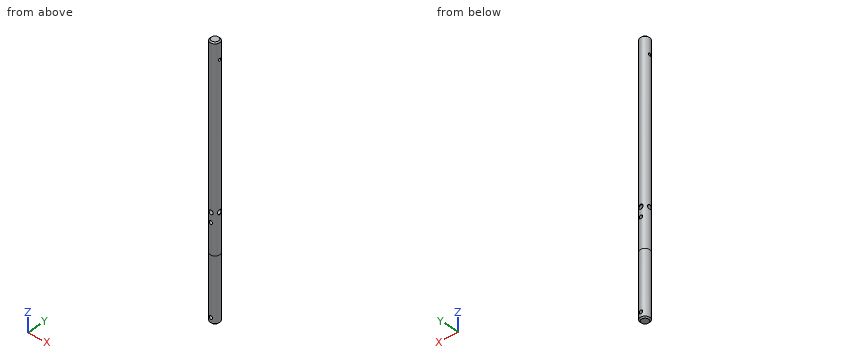
from build123d import *

# Parameters (mm, degrees)
SKETCH1_W                                 = 3.175
SKETCH1_H                                 = 133.223
F_2_56_TAPPED_HOLE1_D                     = 1.778
SKETCH4_R                                 = 3.175
BOSS_EXTRUDE1_DEPTH                       = 43.053
CHAMFER1_SIZE                             = 0.762
F_4_40_TAPPED_HOLE2_D                     = 2.2606
F_7_64_0_10938_DIAMETER_HOLE2_D           = 2.778252
F_7_64_0_10938_DIAMETER_HOLE2_CSINK_D     = 3.175
F_7_64_0_10938_DIAMETER_HOLE2_CSINK_ANGLE = 82


with BuildPart() as part:
    # Sketch1 → Revolve1 (revolve)
    with BuildSketch(Plane.XZ):
        with Locations((1.5875, 66.6115)):
            Rectangle(SKETCH1_W, SKETCH1_H)
    revolve(axis=Axis((0, 0, 133.223), (0, 0, -1)))

    # #2-56 Tapped Hole1 (through all)
    with Locations(Plane(origin=(3.175, 0, 0), x_dir=(0, 0, -1), z_dir=(1, 0, 0))):
        with Locations((-121.801801862, 0)):
            Hole(F_2_56_TAPPED_HOLE1_D / 2)

    # Sketch4 → Boss-Extrude1 (add)
    with BuildSketch(Plane(origin=(0, 0, 0), x_dir=(-1, 0, 0), z_dir=(0, 0, -1))):
        Circle(SKETCH4_R)
    extrude(amount=BOSS_EXTRUDE1_DEPTH)

    # Chamfer1
    chamfer1_edges = [part.edges().sort_by_distance(p)[0] for p in [
        (3.175, 0, -43.053),
        (-3.175, 0, 133.223),
    ]]
    chamfer(chamfer1_edges, length=CHAMFER1_SIZE)

    # #4-40 Tapped Hole2 (through all)
    with Locations(Plane(origin=(0, -3.175, 0), x_dir=(-1, 0, 0), z_dir=(0, -1, 0))):
        with Locations((0, -20.32), (0, 39.0271)):
            Hole(F_4_40_TAPPED_HOLE2_D / 2)

    # Sketch10 → 7/64 (0.10938) Diameter Hole1 (revolve, cut)
    with BuildSketch(Plane(origin=(0, -3.175, 26.67), x_dir=(0, 0, -1), z_dir=(1, 0, 0))):
        Polygon((0, 0), (0, 6.35), (1.5875, 6.35), (1.389126, 6.121796818), (1.389126, 0), align=None)
    revolve(axis=Axis((0, -9.525, 26.67), (0, 1, 0)), mode=Mode.SUBTRACT)

    # 7/64 (0.10938) Diameter Hole2 (through all)
    with Locations(Plane(origin=(3.175, 0, 0), x_dir=(0, 0, -1), z_dir=(1, 0, 0))):
        with Locations((-26.67, 0)):
            CounterSinkHole(F_7_64_0_10938_DIAMETER_HOLE2_D / 2, F_7_64_0_10938_DIAMETER_HOLE2_CSINK_D / 2, counter_sink_angle=F_7_64_0_10938_DIAMETER_HOLE2_CSINK_ANGLE)


solid = part.part
Could you check a few things on this model? Use its own coordinates, in mm. Give positions to 0.01 mm unless a question says otherwise; leave off trailing zeros. Order: outer loops, then holes, each group sorted by start corner. A loop starts at its lowest first (then second) coordinate and runs counter-clockwise, first axis right, second up. Notation, with made-up numbers: M 72.5,6.25 L 105.5,6.25 A17 ccw 105.5,33.25 Z; hole C 36,82.5 d4. An arc over 180 degrees is marked long. One line per question, with ' | ' between items.
1. I'm going to push a flat-ended pin straight in: pin 1 (1.5 mm diameter, centred on y = -2, z = 86, fed in from -X). Where does the tip first touch, or does it pass through?
Results:
pin 1: x = -2.92
2. If I drill on line 1 (Z direction, x = 0, y = 1.5); line 2 (Z direction, x = 0, y = 0.25); line 3 (Z direction, x = 1.75, y = 0.5), over which ranges is the centre line in solid material (lowest first)?
Results:
line 1: -43.05 to -40.16, -37.9 to 19.19, 21.45 to 25.28, 28.06 to 133.22 | line 2: -43.05 to -40.16, -37.9 to 19.19, 21.45 to 25.28, 28.06 to 120.95, 122.65 to 133.22 | line 3: -43.05 to 25.37, 27.97 to 121.07, 122.54 to 133.22
3. I want a section at A-A (z = 111). List the corners of the cut face in (x, y) for me (3 decimals), and give its area (3 significant figures).
Results:
outline: C 0,0 d6.35 | area: 31.7 mm²
